from build123d import *

# Parameters (mm, degrees)
SKETCH2_W                 = 19.05
SKETCH2_H                 = 76.2
BOSS_EXTRUDE2_DEPTH       = 0.508
EDGE_FLANGE2_DEPTH        = 76.2
F_4_CLEARANCE_HOLE1_D     = 3.2639
F_4_CLEARANCE_HOLE1_DEPTH = 0.508


# Sheet-metal steps are written as plain solids
with BuildPart() as part:
    # Sketch2 → Boss-Extrude2 (new body)
    with BuildSketch(Plane(origin=(0, 0, 0), x_dir=(1, 0, 0), z_dir=(0, 1, 0))):
        with Locations((-9.525, 38.1)):
            Rectangle(SKETCH2_W, SKETCH2_H)
    extrude(amount=BOSS_EXTRUDE2_DEPTH)

    # Edge-Flange2 section (across the edge) → Edge-Flange2 (add)
    with BuildSketch(Plane(origin=(5.499261314, 0.508, 0), x_dir=(-0.8660254037844398, -0.499999999999998, 0), z_dir=(0, 0, -1))):
        with BuildLine():
            Line((-0.508, 5.499261314), (-0.508, 57.15))
            Line((-0.508, 57.15), (0, 57.15))
            Line((0, 57.15), (0, 5.499261314))
            ThreePointArc((0, 5.499261314), (1.5875, 2.749630657), (4.7625, 2.749630657))
            Line((4.7625, 2.749630657), (5.0165, 2.309689752))
            ThreePointArc((5.0165, 2.309689752), (1.3335, 2.309689752), (-0.508, 5.499261314))
        make_face()
    extrude(amount=EDGE_FLANGE2_DEPTH)

    # #4 Clearance Hole1
    with Locations(Plane(origin=(0, 0, 0), x_dir=(-1, 0, 0), z_dir=(0, -1, 0))):
        with Locations((6.35, 71.4375), (6.35, 4.7625)):
            Hole(F_4_CLEARANCE_HOLE1_D / 2, depth=F_4_CLEARANCE_HOLE1_DEPTH)


solid = part.part
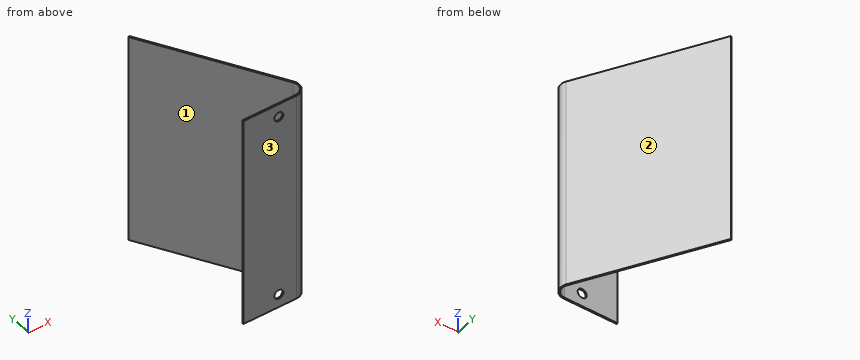
Geometry: final body of the model. Coordinates: model frame, mm. Face numbers are marked on the shaded views. Round coordinates to 2 decimals unless told otherwise and drop trailing zeros. Loops run counter-clockwise (first coordinate to the right, second up) from the corner with the lowest first, then second, coordinate; pieces in that order, holes last. Notation, with made-up numbers: M -35.75,4 L 7.25,4 A30 ccw 7.25,26 Z; hole C 57,33 d1. An arc over 180 degrees is marked long. Put each result on its own line as item: value. Start each with the question number.
(1) Contact query for flat-ended pins moving along their axis: pin 1 Ø15 at (x, z) = (-6.5, -38) entering from +Y; pin 2 Ø2 at (y, z) = (16.5, -37) entering from +X; pin 3 Ø3 at (y, z) = (19.5, -56) entering from -X. Output: stop coordinate, or through.
(2) Draft query along Y for the marked faces 1, 2 and 3. Return one class per face: +Y half, -Y half, draft (parallel to the pull), parting line (faces both ways), or undercut.
(3) Section query C-C (x = -6.35). Return loops of the section in (y, z), then the cut area to 3 significant figures.
(4) Section query D-D (y = 34). Return loops of the section in (x, z), then the cut area to 3 significant figures.
(5) Section query B-B (x = 1.25). Return loops of the section in (y, z).
(6) Material intervals for line 1 along Z through (x, y) = (-6.35, 0.1); line 2 along Y through (x, z) = (1.75, -46); line 3 along Y through (x, z) = (1.5, -62.5), sorted ascending. Write a range as [from, to].
Findings below:
1. pin 1: stops at y = 35.3
1. pin 2: stops at x = -2.57
1. pin 3: stops at x = -6.33
2. face 1: undercut
2. face 2: +Y half
2. face 3: -Y half
3. outline: M 0,-76.2 L 0.51,-76.2 L 0.51,-73.07 L 0,-73.07 Z; M 0,-69.81 L 0.51,-69.81 L 0.51,-6.39 L 0,-6.39 Z; M 0,-3.13 L 0.51,-3.13 L 0.51,0 L 0,0 Z; M 21.03,-76.2 L 22.05,-76.2 L 22.05,0 L 21.03,0 Z
3. area: 113 mm2
4. outline: M -13.84,-76.2 L -13.25,-76.2 L -13.25,0 L -13.84,0 Z
4. area: 44.7 mm2
5. outline: M 0.22,-76.2 L 0.76,-76.2 L 0.76,0 L 0.22,0 Z; M 7.87,-76.2 L 8.88,-76.2 L 8.88,0 L 7.87,0 Z
6. line 1: z = [-76.2, -73.07], [-69.81, -6.39], [-3.13, 0]
6. line 2: y = [0.44, 1.03], [7, 8.02]
6. line 3: y = [0.32, 0.88], [7.43, 8.45]
